The listing builds one solid part. Answer for the finished solid, in the listing's coordinates (mm). A direction names the side the tool comes from. Give positions to 0.01 mm unless a question says otherwise; leave off trailing zeros. Write each loop counter-clockwise with the first axis right and the second up, starting at its lowest first coordinate (ties: lowest second). Pieces come first, ordered by that corner, then holes. Notation, with made-up numbers: M 39,0.5 L 53,0.5 A13 ccw 53,18.5 Z; hole C 87.25,89 d6. An arc over 180 degrees is marked long. Return JSON: item names as keys, results as strings.
from build123d import *

# Parameters (mm, degrees)
SKETCH_1_R      = 2.7
SKETCH_1_R_2    = 1.5
EXTRUDE_1_DEPTH = 2.6
SKETCH_2_R      = 2.7
SKETCH_2_R_2    = 1
EXTRUDE_2_DEPTH = 0.8
SKETCH_3_R      = 3.15
SKETCH_3_R_2    = 1.95
EXTRUDE_3_DEPTH = 2
CHAMFER_1_SIZE  = 0.8


with BuildPart() as part:
    # Эскиз1 → Бобышка-Вытянуть1 (new body)
    with BuildSketch(Plane(origin=(0, 0, 0), x_dir=(1, 0, 0), z_dir=(0, 1, 0))):
        with Locations(Location((0, 0, 0), (0, 0, 270))):
            Circle(SKETCH_1_R)
        with Locations(Location((0, 0, 0), (0, 0, 270))):
            Circle(SKETCH_1_R_2, mode=Mode.SUBTRACT)
    extrude(amount=EXTRUDE_1_DEPTH)

    # Эскиз2 → Бобышка-Вытянуть2 (add)
    with BuildSketch(Plane(origin=(0, 2.6, 0), x_dir=(1, 0, 0), z_dir=(0, 1, 0))):
        with Locations(Location((0, 0, 0), (0, 0, 270))):
            Circle(SKETCH_2_R)
        with Locations(Location((0, 0, 0), (0, 0, 270))):
            Circle(SKETCH_2_R_2, mode=Mode.SUBTRACT)
    extrude(amount=EXTRUDE_2_DEPTH)

    # Эскиз3 → Бобышка-Вытянуть3 (add)
    with BuildSketch(Plane(origin=(0, 3.4, 0), x_dir=(1, 0, 0), z_dir=(0, 1, 0))):
        with Locations(Location((0, 0, 0), (0, 0, 270))):
            Circle(SKETCH_3_R)
        with Locations(Location((0, 0, 0), (0, 0, 270))):
            Circle(SKETCH_3_R_2, mode=Mode.SUBTRACT)
    extrude(amount=EXTRUDE_3_DEPTH)

    # Фаска1
    # the kernel refuses this chamfer: 0.8 mm, written as the material it adds along each edge
    with BuildSketch(Plane(origin=(0, 3.4, 0), x_dir=(0, 0, 1), z_dir=(-1, 0, 0))) as chamfer_1_piece_1_section:
        Polygon((2.7, -CHAMFER_1_SIZE), (2.7 + CHAMFER_1_SIZE, 0), (2.7, 0), align=None)
    chamfer_1_piece_1 = revolve(axis=Axis((0, 3.4, 0), (0, 1, 0)), mode=Mode.PRIVATE)
    chamfer_1_piece_1 = chamfer_1_piece_1 & Plane(origin=(0, 2.825856837, 0), x_dir=(0, 0, 1), z_dir=(0, -1, 0)) * Cylinder(3.15, 14, mode=Mode.PRIVATE)
    add(chamfer_1_piece_1)


solid = part.part
Item 1: A cutting plane is placed at A-A, the plane x = 0. Write down the section's boundary in (y, z).
Geometry results:
{"outline": "M 0,-2.7 L 2.6,-2.7 L 3.05,-3.15 L 5.4,-3.15 L 5.4,-1.95 L 3.4,-1.95 L 3.4,-1 L 2.6,-1 L 2.6,-1.5 L 0,-1.5 Z; M 0,1.5 L 2.6,1.5 L 2.6,1 L 3.4,1 L 3.4,1.95 L 5.4,1.95 L 5.4,3.15 L 3.05,3.15 L 2.6,2.7 L 0,2.7 Z"}
Item 2: Which of the six approach directions +Z, -Z, +X, -X, +Y, -Y give full straight-line access (tool end or side, diameter ignored) to faces 5 (the cylindrical face through (1.917, 4.209, -2.5)), 6 (the flat face through (-1, 3.4, 1))?
Geometry results:
{"face 5": "+Y, -Y", "face 6": "+Y"}
Item 3: A cutting plane is placed at D-D, the plane y = 1.55. Write down the section's boundary in (x, z).
Geometry results:
{"outline": "C 0,0 d5.4; hole C 0,0 d3"}
Item 4: A cutting plane is placed at C-C, the plane y = 4.4. Write down the section's boundary in (x, z), plus the area to 3 significant figures.
Geometry results:
{"outline": "C 0,0 d6.3; hole C 0,0 d3.9", "area": "19.2 mm2"}
Item 5: A cutting plane is placed at B-B, the plane z = 0. Write down the section's boundary in (x, y), plus the area to 3 significant figures.
Geometry results:
{"outline": "M -3.15,3.05 L -2.7,2.6 L -2.7,0 L -1.5,0 L -1.5,2.6 L -1,2.6 L -1,3.4 L -1.95,3.4 L -1.95,5.4 L -3.15,5.4 Z; M 1,2.6 L 1.5,2.6 L 1.5,0 L 2.7,0 L 2.7,2.6 L 3.15,3.05 L 3.15,5.4 L 1.95,5.4 L 1.95,3.4 L 1,3.4 Z", "area": "14.3 mm2"}
Item 6: Given pin 1 Ø2.5 at (x, z) = (0, 0) entering from -Y; pin 2 Ø2.5 at (x, z) = (0, 0) entering from +Y; pin 3 Ø2 at (x, y) = (2.5, 4.5) entering from -Z, each flat-ended and moving along its own axis, determine where each tip first touches the part or whether it passes through.
Geometry results:
{"pin 1": "stops at y = 2.6", "pin 2": "stops at y = 3.4", "pin 3": "stops at z = -2.77"}
Item 7: Determine the mould class of faces 1 (the flat face through (0, 5.4, 2.1)), 2 (the cylindrical face through (-1.187, 4.386, -1.547)), 3 (the cylindrical face through (0.811, 1.282, 2.575)), 4 (the cylindrical face through (0.45, 1.28, 1.43)) for opening direction X: +X half, -X half, draft (parallel to the pull), parting line (faces both ways), or undercut.
Geometry results:
{"face 1": "draft", "face 2": "undercut", "face 3": "parting line", "face 4": "undercut"}
Item 8: Find the intervals of material crossed by line 1 (X direction, y = 0.55, z = 0); line 2 (X direction, y = 0.6, z = -0.5); line 3 (Y direction, x = 1.75, z = 0.25), in increasing order.
Geometry results:
{"line 1": "x = -2.7 to -1.5, 1.5 to 2.7", "line 2": "x = -2.65 to -1.41, 1.41 to 2.65", "line 3": "y = 0 to 3.4"}
